Part model, mm, in its own coordinate system. Coordinates: 2 decimals unless noted, no trailing zeros. Loops run counter-clockwise (first coordinate to the right, second up) from the corner with the lowest first, then second, coordinate; pieces in that order, holes last. Notation, with made-up numbers: (87, 52) -> (121, 52) arc R17 cw to (121, 63) -> close; hole circle Ø6 at (27, 67.25). An arc over 180 degrees is marked (long way). Use one line per item in the form item = value. Start each with the question number.
(1) Drill centre lines: L1, parallel to Y at x = 0, z = -2.5; L2, parallel to X at y = 0.5, z = -0.75; L3, parallel to X at y = -1.5, z = -0.5. Where is each one in solid material? Low to high. Write a range as [from, to].
(2) Mould opens along X. For faces 1 (the flat face through (-2.6, 1.5, 0.1)), 2 (the flat face through (2.6, -1.5, 0.1)), 3 (the cylindrical face through (0, 2, 0)) say: +X half, -X half, draft (parallel to the pull), parting line (faces both ways), or undercut.
(3) Band-saw the part on C-C on z = -2. Give the cut face in (x, y).
(4) Band-saw the part on A-A on y = 0. Give the cut face in (x, z), then the cut area to 3 significant figures.
(5) Band-saw the part on B-B on x = 0. Give the cut face in (y, z), then the cut area to 3 significant figures.
```python
from build123d import *

# Parameters (mm, degrees)
SKETCH4_R           = 2.5
BOSS_EXTRUDE1_DEPTH = 5
SKETCH5_OUTSIDE_W   = 53.21
SKETCH5_OUTSIDE_H   = 52.282
SKETCH5_OUTSIDE_R   = 2.8125
CUT_EXTRUDE1_DEPTH  = 12
CUT_EXTRUDE1_DRAFT  = -60
SKETCH6_OUTSIDE_W   = 53.21
SKETCH6_OUTSIDE_H   = 52.282
SKETCH6_OUTSIDE_R   = 2.8125
CUT_EXTRUDE2_DEPTH  = 12
CUT_EXTRUDE2_DRAFT  = -60
FILLET1_R           = 0.6


with BuildPart() as part:
    # Sketch3 → Revolve1 (revolve)
    with BuildSketch(Plane(origin=(0, 0, 0), x_dir=(0, 0, -1), z_dir=(1, 0, 0)), mode=Mode.PRIVATE) as revolve1_sk:
        Polygon((5, 2.40625), (5, 3), (0, 3), (-5, 3), (-5, 2.40625), (-4.765451453, 2), (4.765451453, 2), align=None)
        Polygon((5, 2.40625), (5, 3), (0, 3), (-5, 3), (-5, 2.40625), (-4.765451453, 2), (4.765451453, 2), align=None)
    revolve(revolve1_sk.sketch.rotate(Axis((0, 0, -5), (0, 0, 1)), 90), axis=Axis((0, 0, -5), (0, 0, 1)))

    # Sketch4 → Boss-Extrude1 (add, symmetric)
    with BuildSketch(Plane.XY):
        Polygon((-1.732050808, 3), (-3.464101615, 0), (-1.732050808, -3), (1.732050808, -3), (3.464101615, 0), (1.732050808, 3), align=None)
        Circle(SKETCH4_R, mode=Mode.SUBTRACT)
    extrude(amount=BOSS_EXTRUDE1_DEPTH, both=True)


with BuildPart() as cut_extrude1_tool:
    # Sketch5 outside → Cut-Extrude1 (with draft: the straight prism first)
    with BuildSketch(Plane.XY.offset(5)):
        Rectangle(SKETCH5_OUTSIDE_W, SKETCH5_OUTSIDE_H)
        Circle(SKETCH5_OUTSIDE_R, mode=Mode.SUBTRACT)
    extrude(amount=-CUT_EXTRUDE1_DEPTH)
    # Cut-Extrude1: the draft: its side faces are tilted about the plane it starts from
    cut_extrude1_sides = [cut_extrude1_tool.faces().sort_by_distance(p)[0] for p in [
        (0, -26.141, -1),
        (26.605, 0, -1),
        (0, 26.141, -1),
        (-26.605, 0, -1),
        (-2.8125, 0, -1),
    ]]
    draft(cut_extrude1_sides, Plane.XY.offset(5), CUT_EXTRUDE1_DRAFT)


with BuildPart() as part_1:
    add(part.part)

    # Cut-Extrude1: cut by cut_extrude1_tool
    add(cut_extrude1_tool.part, mode=Mode.SUBTRACT)


with BuildPart() as cut_extrude2_tool:
    # Sketch6 outside → Cut-Extrude2 (with draft: the straight prism first)
    with BuildSketch(Plane(origin=(0, 0, -5), x_dir=(-1, 0, 0), z_dir=(0, 0, -1))):
        Rectangle(SKETCH6_OUTSIDE_W, SKETCH6_OUTSIDE_H)
        Circle(SKETCH6_OUTSIDE_R, mode=Mode.SUBTRACT)
    extrude(amount=-CUT_EXTRUDE2_DEPTH)
    # Cut-Extrude2: the draft: its side faces are tilted about the plane it starts from
    cut_extrude2_sides = [cut_extrude2_tool.faces().sort_by_distance(p)[0] for p in [
        (0, -26.141, 1),
        (-26.605, 0, 1),
        (0, 26.141, 1),
        (26.605, 0, 1),
        (2.8125, 0, 1),
    ]]
    draft(cut_extrude2_sides, Plane(origin=(0, 0, -5), x_dir=(-1, 0, 0), z_dir=(0, 0, -1)), CUT_EXTRUDE2_DRAFT)


with BuildPart() as part_2:
    add(part_1.part)

    # Cut-Extrude2: cut by cut_extrude2_tool
    add(cut_extrude2_tool.part, mode=Mode.SUBTRACT)

    # Fillet1
    # the kernel refuses this fillet: 0.6 mm, written as the material it takes off along each edge
    with BuildSketch(Plane(origin=(1.732050808, 3, 5.489823036), x_dir=(0.4999999999999995, -0.866025403784439, 0), z_dir=(0, 0, -1)), Plane(origin=(-3.464101615, 0, -5.489823036), x_dir=(0.5000000000000011, -0.8660254037844379, 0), z_dir=(0, 0, 1)), Plane(origin=(3.464101615, 0, 5.489823036), x_dir=(-0.4999999999999996, -0.8660254037844388, 0), z_dir=(0, 0, -1)), Plane(origin=(-1.732050808, 3, 5.489823036), x_dir=(1, 0, 0), z_dir=(0, 0, -1))) as fillet1_piece_1:
        with BuildLine():
            CenterArc((FILLET1_R * 0.57735026919, FILLET1_R), FILLET1_R, 210, 60)
            Line((-FILLET1_R * 0.288675134595, FILLET1_R * 0.5), (0, 0))
            Line((0, 0), (FILLET1_R * 0.57735026919, 0))
        make_face()
    extrude(amount=10.979646072, mode=Mode.SUBTRACT)
    with BuildSketch(Plane(origin=(-1.732050808, -3, -5.489823036), x_dir=(-0.5000000000000002, 0.8660254037844385, 0), z_dir=(0, 0, 1)), Plane(origin=(1.732050808, -3, -5.489823036), x_dir=(-1, 0, 0), z_dir=(0, 0, 1))) as fillet1_piece_2:
        with BuildLine():
            CenterArc((FILLET1_R * 0.57735026919, -FILLET1_R), FILLET1_R, 90, 60)
            Line((-FILLET1_R * 0.288675134595, -FILLET1_R * 0.5), (0, 0))
            Line((0, 0), (FILLET1_R * 0.57735026919, 0))
        make_face()
    extrude(amount=10.979646072, mode=Mode.SUBTRACT)


solid = part_2.part
```
A:
q1.L1 = [-3, -2], [2, 3]
q1.L2 = [-3.18, -1.94], [1.94, 3.18]
q1.L3 = [-2.6, -1.32], [1.32, 2.6]
q2.face_1 = -X half
q2.face_2 = +X half
q2.face_3 = undercut
q3.outline = (-3.29, -0.3) -> (-1.91, -2.7) arc R0.6 ccw to (-1.39, -3) -> (1.39, -3) arc R0.6 ccw to (1.91, -2.7) -> (3.29, -0.3) arc R0.6 ccw to (3.29, 0.3) -> (1.91, 2.7) arc R0.6 ccw to (1.39, 3) -> (-1.39, 3) arc R0.6 ccw to (-1.91, 2.7) -> (-3.29, 0.3) arc R0.6 ccw to start; hole circle Ø4 at (0, 0)
q4.outline = (-3.37, -4.68) -> (-2.81, -5) -> (-2.41, -5) -> (-2, -4.77) -> (-2, 4.77) -> (-2.41, 5) -> (-2.81, 5) -> (-3.37, 4.68) -> close; (2, -4.77) -> (2.41, -5) -> (2.81, -5) -> (3.37, -4.68) -> (3.37, 4.68) -> (2.81, 5) -> (2.41, 5) -> (2, 4.77) -> close
q4.area = 26.9 mm²
q5.outline = (-3, -4.89) -> (-2.81, -5) -> (-2.41, -5) -> (-2, -4.77) -> (-2, 4.77) -> (-2.41, 5) -> (-2.81, 5) -> (-3, 4.89) -> close; (2, -4.77) -> (2.41, -5) -> (2.81, -5) -> (3, -4.89) -> (3, 4.89) -> (2.81, 5) -> (2.41, 5) -> (2, 4.77) -> close
q5.area = 19.8 mm²
